Geometry check sheet. Reference: the model listing, model coordinates, mm. A direction names the side the tool comes from. Coordinates: 2 decimals unless noted, no trailing zeros. Order: outer loops, then holes, each group sorted by start corner. A loop starts at its lowest first (then second) coordinate and runs counter-clockwise, first axis right, second up. Notation, with made-up numbers: (22.5, 13.25) - (74.5, 13.25) arc R10 ccw to (74.5, 23.25) - close; hole circle Ø6 at (-32, 2). An arc over 180 degrees is marked (long way). Use CSV: the item, a comma, the result in double quotes. Start each with the question number.
1) Sectioned sample at D-D, the plane y = 15.5. Record the cut outline in (x, z), and give its area (3 significant figures).
2) Sectioned sample at A-A, the plane y = 2. Record the cut outline in (x, z).
3) Sectioned sample at B-B, the plane x = 2. Record the cut outline in (y, z), and give its area (3 significant figures).
4) Depth check by flat-ended pin: P1, Ø3, axis at x = -16, y = 6, coming from the +Z side. Enter the tip coordinate at first touch or a pass-through.
5) Thickness scan on probe 1 along Z at (x, y) = (12, 10.5). Record the ranges inside material, lowest first. Write a range as [from, to].
6) Tool access check on faces 1 (the cylindrical face through (1.2, 1.4, 11)), 2 (the flat face through (0, 20, 5)). Record the directions out of +Z, -Z, +X, -X, +Y, -Y that give a thin tool (end or side, any length) a straight path to the whole face; none if there is none.
7) Sectioned sample at C-C, the plane z = 11. Record the cut outline in (x, y).
from build123d import *

# Parameters (mm, degrees)
SKETCH_1_W     = 20
SKETCH_1_H     = 20
BASEBOX_DEPTH  = 10
SKETCH_2_R     = 1
BOSSSEED_DEPTH = 2


with BuildPart() as part:
    # 草图1 → BaseBox (new body)
    with BuildSketch(Plane.XY):
        with Locations((10, 10)):
            Rectangle(SKETCH_1_W, SKETCH_1_H)
    basebox = extrude(amount=BASEBOX_DEPTH)

    # 草图2 → BossSeed (add)
    with BuildSketch(Plane.XY.offset(10)):
        with Locations((2, 2)):
            Circle(SKETCH_2_R)
    extrude(amount=BOSSSEED_DEPTH)

    # Mirror 2: BaseBox across plane
    add(basebox.mirror(Plane(origin=(0, 0, 0), x_dir=(0, 0, 1), z_dir=(1, 0, 0))))


solid = part.part
Evaluation:
1,outline,"(-20, 0) - (20, 0) - (20, 10) - (-20, 10) - close"
1,area,"400 mm²"
2,outline,"(-20, 0) - (20, 0) - (20, 10) - (3, 10) - (3, 12) - (1, 12) - (1, 10) - (-20, 10) - close"
3,outline,"(0, 0) - (20, 0) - (20, 10) - (3, 10) - (3, 12) - (1, 12) - (1, 10) - (0, 10) - close"
3,area,"204 mm²"
4,P1,"z = 10"
5,probe 1,"[0, 10]"
6,face 1,"+Z"
6,face 2,"+Z, -Z, +X, -X, +Y"
7,outline,"circle Ø2 at (2, 2)"
